from build123d import *

# Parameters (mm, degrees)
SKETCH_3_R          = 7
EXTRUDE_1_DEPTH     = 1
EXTRUDE_START       = 1
SKETCH_4_R          = 7
EXTRUDE_2_DEPTH     = 1
SKETCH_5_R          = 3
CUT_EXTRUDE_3_DEPTH = 12.090536506
FILLET_2_R          = 1
FILLET_3_R          = 1


with BuildPart() as part:
    # Эскиз2 → Повернуть1 (revolve)
    with BuildSketch(Plane(origin=(0, 0, 0), x_dir=(1, 0, 0), z_dir=(0, 1, 0))):
        Polygon((7, 0), (0, 0), (0, 3), (7, 3), (6, 1.5), align=None)
    revolve(axis=Axis((0, 0, 0), (0, 0, -1)))

    # Эскиз3 → Вытянуть1 (add)
    with BuildSketch(Plane(origin=(0, 0, -3), x_dir=(-1, 0, 0), z_dir=(0, 0, -1))):
        Circle(SKETCH_3_R)
    extrude(amount=EXTRUDE_1_DEPTH)

    # Эскиз4 → Вытянуть2 (add)
    with BuildSketch(Plane.XY.offset(EXTRUDE_START)):
        with Locations(Location((0, 0, 0), (0, 0, 180))):
            Circle(SKETCH_4_R)
    extrude(amount=-EXTRUDE_2_DEPTH)

    # Эскиз5 → Вытянуть3 (cut, through all)
    with BuildSketch(Plane(origin=(0, 0, -4), x_dir=(-1, 0, 0), z_dir=(0, 0, -1))):
        Circle(SKETCH_5_R)
    extrude(amount=-CUT_EXTRUDE_3_DEPTH, mode=Mode.SUBTRACT)

    # Скругление2
    fillet_2_edges = [part.edges().sort_by_distance(p)[0] for p in [
        (-6, 0, -1.5),
    ]]
    fillet(fillet_2_edges, radius=FILLET_2_R)

    # Скругление3
    fillet_3_edges = [part.edges().sort_by_distance(p)[0] for p in [
        (3, 0, 1),
        (3, 0, -4),
    ]]
    fillet(fillet_3_edges, radius=FILLET_3_R)


solid = part.part
Work out the finished part from the listing and answer in its coordinate system (mm). Round coordinates to 2 decimals unless told otherwise and drop trailing zeros. Write each loop counter-clockwise with the first axis right and the second up, starting at its lowest first coordinate (ties: lowest second). Pieces come first, ordered by that corner, then holes. Notation, with made-up numbers: (-9.5, -19) -> (-3.5, -19) arc R17 cw to (-3.5, -9) -> close; hole circle Ø9 at (70, 79.5). An arc over 180 degrees is marked (long way). Write each question's results on one line, items separated by ' | '.
Item 1: Find the intervals of material crossed by line 1 along Y through (x, z) = (0, -1.9); line 2 along Y through (x, z) = (2, -3.2); line 3 along X through (y, z) = (-2, 0.8), in increasing order. Write a range as [from, to].
Result set:
line 1: [-6.29, -3], [3, 6.29] | line 2: [-6.71, -2.26], [2.26, 6.71] | line 3: [-6.71, -2.75], [2.75, 6.71]
Item 2: The mould has two halves that part along X. Classify faces 1 (the face through (-3, 3, 1)), 2 (the face through (3, 0, -2)), 3 (the face through (-6.466, -2.681, -3.493)): +X half, -X half, draft (parallel to the pull), parting line (faces both ways), or undercut.
Result set:
face 1: draft | face 2: undercut | face 3: parting line
Item 3: A cutting plane is placed at A-A, the plane z = 0.45. Determine the outline of the cut face in (x, y), plus the area to 3 significant figures.
Result set:
outline: circle Ø14 at (0, 0); hole circle Ø6.21 at (0, 0) | area: 124 mm^2
Item 4: A cutting plane is placed at B-B, the plane z = -2.3. Determine the outline of the cut face in (x, y).
Result set:
outline: circle Ø13.07 at (0, 0); hole circle Ø6 at (0, 0)
Item 5: Flat-ended cylindrical pins translate along their axes: P1, Ø1.5, axis at y = -1, z = -2.5, coming from the +X side; P2, Ø1, axis at x = -5, z = -2.5, coming from the +Y side; P3, Ø1, axis at y = -2, z = -1.5, coming from the +X side; P4, Ø4, axis at x = -5, y = 5, coming from the -Z side. Find the tip coordinate at first contact, or state that the pin passes through.
Result set:
P1: x = 6.99 | P2: y = 5.1 | P3: x = 6.05 | P4: z = -4
